from build123d import *

# Parameters (mm, degrees)
BOSS_EXTRUDE1_DEPTH      = 12.7
CUT_EXTRUDE1_START       = -12.7
CUT_EXTRUDE1_OUTLINE_R   = 5
CUT_EXTRUDE1_OUTLINE_R_2 = 1.85
CUT_EXTRUDE1_DEPTH       = 12.7
SKETCH5_R                = 5
SKETCH5_R_2              = 1.85
CUT_EXTRUDE2_DEPTH       = 168.267151587


# Read off the part's stored shape, not the designer's step: Cut-Extrude1
with BuildPart() as part:
    # Sketch1 → Boss-Extrude1 (new body)
    with BuildSketch(Plane(origin=(0, 0, 0), x_dir=(0, 0, -1), z_dir=(1, 0, 0))):
        with BuildLine():
            ThreePointArc((-4.073644652, -24.665875603), (25, 0), (-4.073644652, 24.665875603))
            ThreePointArc((-4.073644652, 24.665875603), (-77.987776172, 15.546567094), (-152.4, 12.5))
            ThreePointArc((-152.4, 12.5), (-164.9, 0), (-152.4, -12.5))
            ThreePointArc((-152.4, -12.5), (-77.987776172, -15.546567094), (-4.073644652, -24.665875603))
        make_face()
    extrude(amount=BOSS_EXTRUDE1_DEPTH)

    # Cut-Extrude1 outline → Cut-Extrude1 (cut)
    with BuildSketch(Plane(origin=(12.7, 0, 0), x_dir=(0, 0, -1), z_dir=(1, 0, 0)).offset(CUT_EXTRUDE1_START)):
        Circle(CUT_EXTRUDE1_OUTLINE_R)
        with Locations((13.029498672, 13.274798425)):
            Circle(CUT_EXTRUDE1_OUTLINE_R_2)
        with Locations((13.029498672, -13.274798425)):
            Circle(CUT_EXTRUDE1_OUTLINE_R_2)
        with Locations((-13.029498672, -13.274798425)):
            Circle(CUT_EXTRUDE1_OUTLINE_R_2)
        with Locations((-13.029498672, 13.274798425)):
            Circle(CUT_EXTRUDE1_OUTLINE_R_2)
    extrude(amount=CUT_EXTRUDE1_DEPTH, mode=Mode.SUBTRACT)

    # Sketch5 → Cut-Extrude2 (cut, through all)
    with BuildSketch(Plane(origin=(12.7, 0, 0), x_dir=(0, 0, -1), z_dir=(1, 0, 0))):
        with Locations((-152.4, 0)):
            Circle(SKETCH5_R)
        with Locations((-143.9, 0)):
            Circle(SKETCH5_R_2)
        with Locations((-152.4, -8.5)):
            Circle(SKETCH5_R_2)
        with Locations((-160.9, 0)):
            Circle(SKETCH5_R_2)
        with Locations((-152.4, 8.5)):
            Circle(SKETCH5_R_2)
        with Locations((-133.9, 0)):
            Circle(SKETCH5_R_2)
        with Locations((-123.9, 0)):
            Circle(SKETCH5_R_2)
    extrude(amount=-CUT_EXTRUDE2_DEPTH, mode=Mode.SUBTRACT)


solid = part.part
Geometry check sheet. Reference: the model listing, model coordinates, mm. Coordinates: 2 decimals unless noted, no trailing zeros. Order: outer loops, then holes, each group sorted by start corner. A loop starts at its lowest first (then second) coordinate and runs counter-clockwise, first axis right, second up. Notation, with made-up numbers: (-4.75, 53) - (31.25, 53) arc R21 cw to (31.25, 79) - close; hole circle Ø9 at (60.5, 42.5). An arc over 180 degrees is marked (long way). Answer in a Markdown table with one row per item. Add a question column.
1) Gauge pin test, flat ends, axial feed: P1, Ø5, axis at x = 5.5, y = 7, coming from the +Z side; P2, Ø9, axis at y = 0, z = 0, coming from the +X side; P3, Ø1.5, axis at x = 6, z = 144, coming from the -Y side; P4, Ø1, axis at x = 11, z = 107, coming from the +Y side. Record the tip position at first contact, or that the pin passes through.
2) Cross-section at C-C, the plane x = 6.25. State how many separate pieces and enclosed holes the cut face has, then the cut area to 3 significant figures.
3) Cross-section at A-A, the plane z = 0. Record the cut outline in (x, y).
4) Release check for a two-part mould opening along Y. For faces 1 (the cylindrical face through (6.261, -0.607, -24.993)), 2 (the cylindrical face through (6.26, 14.83, 12.03)), 3 (the cylindrical face through (6.261, 15.632, 76.948)) record: +Y half, -Y half, draft (parallel to the pull), parting line (faces both ways), or undercut.
5) Cross-section at D-D, the plane z = 76. Record the cut outline in (x, y).
6) Cross-section at B-B, the plane y = 8.5. Record the cut outline in (x, z), then the cut area to 3 significant figures.
7) Material ranges on line 1 along Y through (x, z) = (3.25, 0); line 2 along Z through (x, y) = (0.5, -2); line 3 along Z through (x, y) = (1, 3), recorded low to high. Write a range as [from, to].
Check result:
| question | item | result |
|---|---|---|
| 1 | P1 | stops at z = 164.06 |
| 1 | P2 | passes through |
| 1 | P3 | stops at y = -12.55 |
| 1 | P4 | stops at y = 13.66 |
| 2 | separate pieces | 1 |
| 2 | enclosed holes | 12 |
| 2 | area | 6,070 mm² |
| 3 | outline | (0, -25) - (12.7, -25) - (12.7, -5) - (0, -5) - close; (0, 5) - (12.7, 5) - (12.7, 25) - (0, 25) - close |
| 4 | face 1 | parting line |
| 4 | face 2 | undercut |
| 4 | face 3 | +Y half |
| 5 | outline | (0, -15.71) - (12.7, -15.71) - (12.7, 15.71) - (0, 15.71) - close |
| 6 | outline | (0, -23.51) - (12.7, -23.51) - (12.7, 150.55) - (0, 150.55) - close; (0, 154.25) - (12.7, 154.25) - (12.7, 161.57) - (0, 161.57) - close |
| 6 | area | 2,300 mm² |
| 7 | line 1 | y = [-25, -5], [5, 25] |
| 7 | line 2 | z = [-24.92, -4.58], [4.58, 147.82], [156.98, 164.74] |
| 7 | line 3 | z = [-24.82, -4], [4, 148.4], [156.4, 164.53] |
